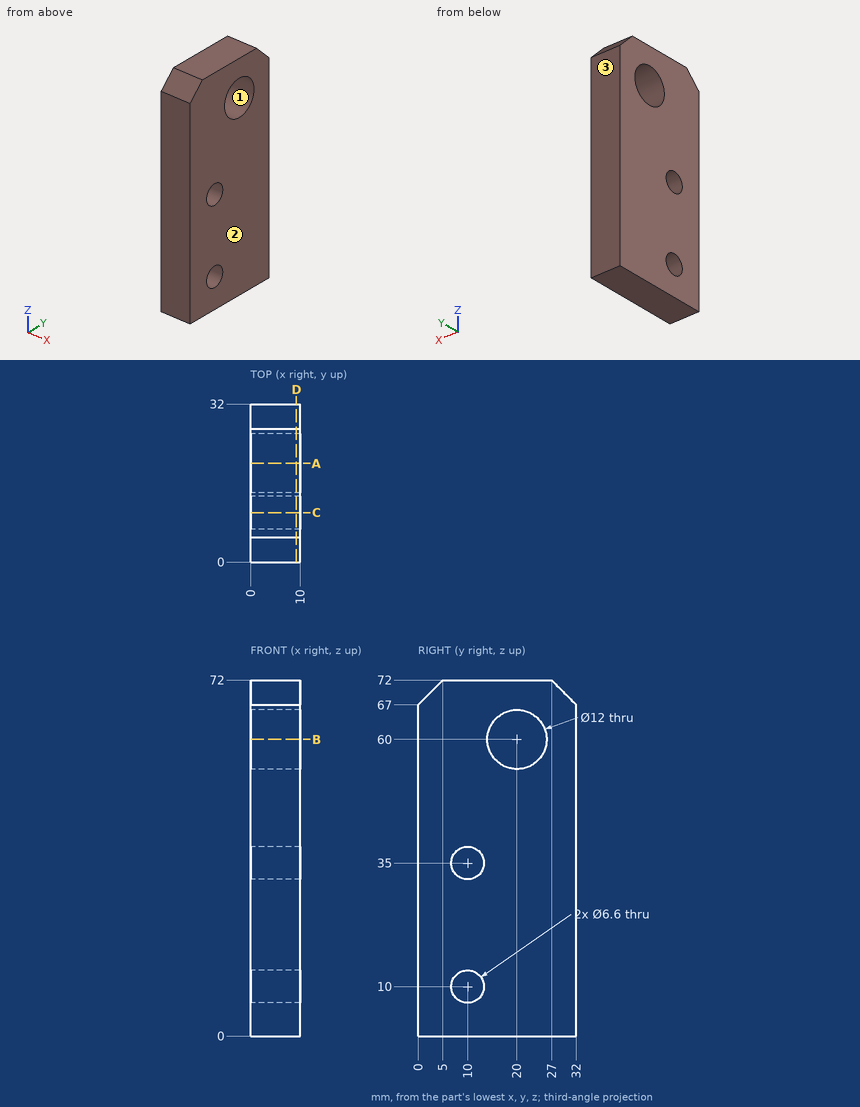
Answer from the drawing. Dimensions are ordinates in mm from the lowest x, y and z of the part. Give positions to 0.01 mm unless a question says otherwise; leave off trailing zeros. Write each loop counter-clockwise with the first axis right and the second up, starting at its lowest first coordinate (ties: lowest second). Pieces come first, ordered by that corner, then holes. Notation, with made-up numbers: (15.5, -24) -> (42.5, -24) arc R15 cw to (42.5, -2) -> close; hole circle Ø4 at (50.5, 27.5). An arc over 180 degrees is marked (long way). Use a Markdown table: item, result.
(1) Section C-C, the plane y = 10 is taken. Determine the outline of the cut face in (x, z).
Return value:
| item | result |
|---|---|
| outline | (0, 0) -> (10, 0) -> (10, 6.7) -> (0, 6.7) -> close; (0, 13.3) -> (10, 13.3) -> (10, 31.7) -> (0, 31.7) -> close; (0, 38.3) -> (10, 38.3) -> (10, 72) -> (0, 72) -> close |
(2) Section A-A, the plane y = 20 is taken. Determine the outline of the cut face in (x, z), then the cut area to 3 significant figures.
Return value:
| item | result |
|---|---|
| outline | (0, 0) -> (10, 0) -> (10, 54) -> (0, 54) -> close; (0, 66) -> (10, 66) -> (10, 72) -> (0, 72) -> close |
| area | 600 mm2 |
(3) A flat-ended cylindrical pin translates along its axis: P1, Ø4, axis at y = 10, z = 35, coming from the +X side. Find the tip coordinate at first contact, or state that the pin passes through.
Return value:
| item | result |
|---|---|
| P1 | through |
(4) Determine the mould class of the marked faces 1, 2 and 3 for opening direction Y: released by +Y, released by -Y, zero draft, split by the parting line, or undercut.
Return value:
| item | result |
|---|---|
| face 1 | undercut |
| face 2 | zero draft |
| face 3 | released by +Y |
(5) Section D-D, the plane x = 9.25 is taken. Determine the outline of the cut face in (y, z).
Return value:
| item | result |
|---|---|
| outline | (0, 0) -> (32, 0) -> (32, 67) -> (27, 72) -> (5, 72) -> (0, 67) -> close; hole circle Ø6.6 at (10, 10); hole circle Ø6.6 at (10, 35); hole circle Ø12 at (20, 60) |
(6) Section B-B, the plane z = 60 is taken. Determine the outline of the cut face in (x, y).
Return value:
| item | result |
|---|---|
| outline | (0, 0) -> (10, 0) -> (10, 14) -> (0, 14) -> close; (0, 26) -> (10, 26) -> (10, 32) -> (0, 32) -> close |
(7) Find the intervals of material crossed by probe 1 along Z at (x, y) = (6, 10); probe 2 along Z at (x, y) = (6, 20); probe 3 along Z at (x, y) = (7.75, 13), in increasing order. Write a range as from..to.
Return value:
| item | result |
|---|---|
| probe 1 | 0..6.7, 13.3..31.7, 38.3..72 |
| probe 2 | 0..54, 66..72 |
| probe 3 | 0..8.63, 11.37..33.63, 36.37..72 |
